Source: CAD feature listing. Evaluate the final solid. Frame: model axes, mm. A direction names the side the tool comes from. Give positions to 0.01 mm unless a question says otherwise; leave off trailing zeros. Write each loop counter-clockwise with the first axis right and the second up, starting at its lowest first coordinate (ties: lowest second). Pieces come first, ordered by that corner, then holes.
Autodesk Inventor part; units mm, degrees
ref_plane "YZ Plane" through (0, 0, 0) normal (1, 0, 0) x (0, 1, 0)
ref_plane "XZ Plane" through (0, 0, 0) normal (0, 1, 0) x (-1, 0, 0)
ref_plane "XY Plane" through (0, 0, 0) normal (0, 0, 1) x (1, 0, 0)
sketch "Sketch1" plane through (0, 0, 0) normal (0, 1, 0) x (-1, 0, 0)
  line L0 (53.975, 0) -> (250.825, 0)
  line L1 (304.8, -53.975) -> (304.8, -1470.025)
  line L2 (250.825, -1524) -> (53.975, -1524)
  line L3 (0, -1470.025) -> (0, -53.975)
  circle A0 centre (263.525, -41.275) radius 5.5563
  circle A1 centre (263.525, -762) radius 5.5563
  circle A2 centre (263.525, -1482.725) radius 5.5563
  circle A3 centre (41.275, -41.275) radius 5.5563
  circle A4 centre (41.275, -762) radius 5.5563
  circle A5 centre (41.275, -1482.725) radius 5.5563
  arc A6 (304.8, -53.975) -> (250.825, 0) centre (250.825, -53.975) ccw
  arc A7 (0, -1470.025) -> (53.975, -1524) centre (53.975, -1470.025) ccw
  arc A8 (250.825, -1524) -> (304.8, -1470.025) centre (250.825, -1470.025) ccw
  arc A9 (53.975, 0) -> (0, -53.975) centre (53.975, -53.975) ccw
  point P0 (0, 0)
  point P1 (304.8, -1524)
  point P2 (0, -1524)
  dimension "d0" = 304.8
  dimension "d1" = 1524
  dimension "d2" = 11.1125
  dimension "d5" = 720.725
  dimension "d8" = 222.25
  dimension "d11" = 41.275
  dimension "d12" = 41.275
  dimension "d13" = 53.975
extrude "Extrusion1" add sketch "Sketch1" along normal blind 22.225
ref_plane "Work Plane3" through (0, 17.4625, 0) normal (0, 1, 0) x (1, 0, 0)
sketch "Sketch2" plane through (0, 17.4625, 0) normal (0, 1, 0) x (1, 0, 0)
  circle A0 centre (-41.275, 1482.725) radius 5.5562
  circle A1 centre (-41.275, 762) radius 5.5562
  circle A2 centre (-41.275, 41.275) radius 5.5562
  circle A3 centre (-263.525, 1482.725) radius 5.5562
  circle A4 centre (-263.525, 762) radius 5.5562
  circle A5 centre (-263.525, 41.275) radius 5.5562
  line L0 (-250.825, 0) -> (-53.975, 0)
  arc A6 (-53.975, 0) -> (0, 53.975) centre (-53.975, 53.975) ccw
  line L1 (0, 53.975) -> (0, 1470.025)
  arc A7 (0, 1470.025) -> (-53.975, 1524) centre (-53.975, 1470.025) ccw
  line L2 (-53.975, 1524) -> (-250.825, 1524)
  arc A8 (-250.825, 1524) -> (-304.8, 1470.025) centre (-250.825, 1470.025) ccw
  line L3 (-304.8, 1470.025) -> (-304.8, 53.975)
  arc A9 (-304.8, 53.975) -> (-250.825, 0) centre (-250.825, 53.975) ccw
  line L4 (0, 53.975) -> (0, 1470.025)
  arc A10 (-250.825, 1524) -> (-304.8, 1470.025) centre (-250.825, 1470.025) ccw
  line L5 (-53.975, 1524) -> (-250.825, 1524)
  line L6 (-304.8, 1470.025) -> (-304.8, 53.975)
  line L7 (-304.8, 1470.025) -> (-304.8, 53.975)
  line L8 (-250.825, 0) -> (-53.975, 0)
  point P0 (0, 0)
ref_plane "Work Plane4" through (0, 4.7625, 0) normal (0, -1, 0) x (1, 0, 0)
sketch "Sketch3" plane through (0, 4.7625, 0) normal (0, -1, 0) x (1, 0, 0)
  circle A0 centre (-41.275, -1482.725) radius 5.5562
  circle A1 centre (-41.275, -762) radius 5.5562
  circle A2 centre (-41.275, -41.275) radius 5.5562
  circle A3 centre (-263.525, -1482.725) radius 5.5562
  circle A4 centre (-263.525, -762) radius 5.5562
  circle A5 centre (-263.525, -41.275) radius 5.5562
  line L0 (-250.825, 0) -> (-53.975, 0)
  arc A6 (0, -53.975) -> (-53.975, 0) centre (-53.975, -53.975) ccw
  line L1 (0, -53.975) -> (0, -1470.025)
  arc A7 (-53.975, -1524) -> (0, -1470.025) centre (-53.975, -1470.025) ccw
  line L2 (-53.975, -1524) -> (-250.825, -1524)
  arc A8 (-304.8, -1470.025) -> (-250.825, -1524) centre (-250.825, -1470.025) ccw
  line L3 (-304.8, -1470.025) -> (-304.8, -53.975)
  arc A9 (-250.825, 0) -> (-304.8, -53.975) centre (-250.825, -53.975) ccw
  line L4 (-299.72, -53.975) -> (-299.72, -1470.025)
  arc A10 (-299.72, -1470.025) -> (-250.825, -1518.92) centre (-250.825, -1470.025) ccw
  line L5 (-250.825, -1518.92) -> (-53.975, -1518.92)
  arc A11 (-53.975, -1518.92) -> (-5.08, -1470.025) centre (-53.975, -1470.025) ccw
  line L6 (-5.08, -1470.025) -> (-5.08, -53.975)
  arc A12 (-5.08, -53.975) -> (-53.975, -5.08) centre (-53.975, -53.975) ccw
  line L7 (-53.975, -5.08) -> (-250.825, -5.08)
  arc A13 (-250.825, -5.08) -> (-299.72, -53.975) centre (-250.825, -53.975) ccw
  point P0 (0, 0)
  dimension "d26" = 5.08
sketch "Sketch8" plane through (0, 22.225, 0) normal (0, 1, 0) x (1, 0, 0)
  arc A0 (-53.975, 0) -> (0, 53.975) centre (-53.975, 53.975) ccw
  line L0 (-250.825, 0) -> (-53.975, 0)
  line L1 (-53.975, 0) -> (-250.825, 0)
  arc A1 (-304.8, 53.975) -> (-250.825, 0) centre (-250.825, 53.975) ccw
  arc A2 (-250.825, 1524) -> (-304.8, 1470.025) centre (-250.825, 1470.025) ccw
  line L2 (-304.8, 53.975) -> (-304.8, 1470.025)
  line L3 (-53.975, 1524) -> (-250.825, 1524)
  line L4 (-250.825, 1524) -> (-53.975, 1524)
  arc A3 (0, 1470.025) -> (-53.975, 1524) centre (-53.975, 1470.025) ccw
  line L5 (0, 1470.025) -> (0, 53.975)
  arc A4 (-53.975, 0) -> (0, 53.975) centre (-53.975, 53.975) ccw
  arc A5 (-304.8, 53.975) -> (-250.825, 0) centre (-250.825, 53.975) ccw
  arc A6 (-250.825, 1524) -> (-304.8, 1470.025) centre (-250.825, 1470.025) ccw
  arc A7 (0, 1470.025) -> (-53.975, 1524) centre (-53.975, 1470.025) ccw
  line L6 (-299.72, 1470.025) -> (-299.72, 53.975)
  arc A8 (-299.72, 53.975) -> (-250.825, 5.08) centre (-250.825, 53.975) ccw
  line L7 (-250.825, 5.08) -> (-53.975, 5.08)
  arc A9 (-53.975, 5.08) -> (-5.08, 53.975) centre (-53.975, 53.975) ccw
  line L8 (-5.08, 53.975) -> (-5.08, 1470.025)
  arc A10 (-5.08, 1470.025) -> (-53.975, 1518.92) centre (-53.975, 1470.025) ccw
  line L9 (-53.975, 1518.92) -> (-250.825, 1518.92)
  arc A11 (-250.825, 1518.92) -> (-299.72, 1470.025) centre (-250.825, 1470.025) ccw
  point P0 (0, 0)
  dimension "d25" = 5.08
extrude "Extrusion2" cut sketch "Sketch3" against normal blind 12.7 contours L0 A6 L1 A7 L2 A8 L3 A9
properties part number "EtgSignModV2"
1. Pull-direction query (Y, two-part tool) for faces 6 (the cylindrical face through (-288.57, 19.81, -15.39)), 7 (the cylindrical face through (-285.777, 11.024, -1504.217)), 8 (the flat face through (-150, 22.225, -751)); classes: pulls with the +Y half, pulls with the -Y half, needs draft (parallel to the pull), parting line crosses it, or undercut.
2. Line query: probe 1 along X at (y, z) = (12.5, -762); probe 2 along Z at (x, y) = (-258.5, 15.5); probe 3 along X at (y, z) = (15, -377). Output: solid intervals per line, ascending.
3. Access query for faces 1 (the cylindrical face through (-285.017, 11.024, -19.023)), 2 (the cylindrical face through (-19.783, 11.024, -1504.977)), 3 (the flat face through (-150, 0, -751)), 4 (the cylindrical face through (-289.41, 19.81, -1507.77)), 5 (the cylindrical face through (-19.023, 11.024, -19.783)). Directions: +Z, -Z, +X, -X, +Y, -Y. A direction counts if a zero-diameter tool reaches every point of the face in a straight line with its end or side. Return the directions, or none.
4. Pin query (flat end, axial travel): P1, Ø6.5, axis at x = -41.275, z = -762, coming from the -Y side; P2, Ø1.5, axis at y = 16.5, z = -530, coming from the +X side; P3, Ø1, axis at y = 9, z = -702, coming from the -X side; P4, Ø4, axis at x = -133.5, y = 12.5, coming from the +Z side. Return the tip coordinate at first contact, or that it passes through.
5. Section query B-B (z = -141.5). Return loops of the section in (x, y) (1 decimal).
6. Section query A-A (y = 9.25). Return loops of the section in (x, z) (3 decimals), plus the area to 3 significant figures.
The answers:
1. face 6: needs draft
1. face 7: undercut
1. face 8: pulls with the +Y half
2. probe 1: x = -299.72 to -269.08, -257.97 to -46.83, -35.72 to -5.08
2. probe 2: z = -1518.31 to -1485.1, -1480.35 to -764.37, -759.63 to -43.65, -38.9 to -5.69
2. probe 3: x = -299.72 to -5.08
3. face 1: +Z, -X
3. face 2: -Z, +X
3. face 3: +Z, -Z, +X, -X, -Y
3. face 4: -Z, -X, +Y, -Y
3. face 5: +Z, +X
4. P1: passes through
4. P2: stops at x = -5.08
4. P3: stops at x = -299.72
4. P4: stops at z = -5.08
5. outline: (-304.8, 0) - (0, 0) - (0, 4.8) - (-5.1, 4.8) - (-5.1, 17.5) - (0, 17.5) - (0, 22.2) - (-304.8, 22.2) - (-304.8, 17.5) - (-299.7, 17.5) - (-299.7, 4.8) - (-304.8, 4.8) - close
6. outline: (-299.72, -1470.025) arc R48.895 ccw to (-250.825, -1518.92) - (-53.975, -1518.92) arc R48.895 ccw to (-5.08, -1470.025) - (-5.08, -53.975) arc R48.895 ccw to (-53.975, -5.08) - (-250.825, -5.08) arc R48.895 ccw to (-299.72, -53.975) - close; hole circle Ø11.113 at (-263.525, -1482.725); hole circle Ø11.113 at (-263.525, -762); hole circle Ø11.113 at (-263.525, -41.275); hole circle Ø11.113 at (-41.275, -1482.725); hole circle Ø11.113 at (-41.275, -762); hole circle Ø11.113 at (-41.275, -41.275)
6. area: 443,000 mm2
